from build123d import *

# Parameters (mm, degrees)
F1_DEPTH = 20
F2_SIZE2 = 9.99999
F2_SIZE  = 9.99999


# Not quite as in the source:
# - a fillet or chamfer is up to 0.001 mm smaller than in the source, because OpenCascade refuses the exact size


with BuildPart() as f1:
    # F0 (on Top) → F1 (new body)
    with BuildSketch(Plane.XY):
        Polygon((-50.6066017178, 10.6066017178), (-40, 0), (-40, -79.367487377), (40, -79.367487377), (40, 0), (50.6066017178, 10.6066017178), (0, 61.2132034356), align=None)
        Polygon((40, -79.367487377), (-40, -79.367487377), (-40, -158.7349747541), (-50.6066017178, -169.3415764719), (0, -219.9481781897), (50.6066017178, -169.3415764719), (40, -158.7349747541), align=None)
    extrude(amount=F1_DEPTH)

    # F2 (size 10 and 10 in the source; OpenCascade refuses exactly that, so slightly less here)
    f2_edges = [f1.edges().sort_by_distance(p)[0] for p in [
        (40, -79.367487, 20),
        (25.303301, 35.909903, 20),
        (-25.303301, 35.909903, 20),
        (-45.303301, 5.303301, 20),
        (45.303301, 5.303301, 20),
        (-40, -79.367487, 20),
        (-45.303301, -164.038276, 20),
        (-25.303301, -194.644877, 20),
        (25.303301, -194.644877, 20),
        (45.303301, -164.038276, 20),
        (40, -79.367487, 0),
        (25.303301, -194.644877, 0),
        (45.303301, -164.038276, 0),
        (-25.303301, -194.644877, 0),
        (-45.303301, -164.038276, 0),
        (-40, -79.367487, 0),
        (-45.303301, 5.303301, 0),
        (-25.303301, 35.909903, 0),
    ]]
    chamfer(f2_edges, length=F2_SIZE, length2=F2_SIZE2)


solid = f1.part
Check sheet for the modelled part. Datum: model origin and axes. Units: mm. A direction names the side the tool comes from. Round coordinates to 2 decimals unless told otherwise and drop trailing zeros. Loops run counter-clockwise (first coordinate to the right, second up) from the corner with the lowest first, then second, coordinate; pieces in that order, holes last. Notation, with made-up numbers: (68, -13) - (108, -13) arc R36 cw to (108, 26) - close; hole circle Ø8 at (15, 87). An arc over 180 degrees is marked (long way). Answer as CSV lines item,"result". Start each with the question number.
Item 1: Section check B-B (z = 14). Record the boundary of the cut face in (x, y), and give its area (3 significant figures).
Item 2: Depth check by flat-ended pin: P1, Ø4, axis at y = -3.5, z = 7, coming from the -X side; P2, Ø2, axis at x = -14, z = 15, coming from the -Y side; P3, Ø1, axis at x = -4, z = 11, coming from the -Y side. Enter the tip coordinate at first touch or a pass-through.
Item 3: Set-up check for faces 1 (the flat face through (-40.159, -166.064, 15.07)), 2 (the flat face through (-38.84, 6.01, 4.93)), 3 (the flat face through (35, -81, 15)): record each of +Z, -Z, +X, -X, +Y, -Y from which the full face is reachable in a straight line by a thin tool's end or side.
Item 4: Scan lines: line 1 (Y direction, x = 42.5, z = 9.5); line 2 (Y direction, x = -19, z = 2.5); line 3 (Z direction, x = 30.5, y = -120). Record each from-to range of solid material in increasing order. Write a range as [from, to].
Report:
1,outline,"(-44.95, -169.34) - (0, -214.29) - (44.95, -169.34) - (36, -160.39) - (36, 1.66) - (44.95, 10.61) - (0, 55.56) - (-44.95, 10.61) - (-36, 1.66) - (-36, -160.39) - close"
1,area,"17,200 mm2"
2,P1,"stops at x = -39"
2,P2,"stops at y = -200.61"
2,P3,"stops at y = -215.4"
3,face 1,"+Z, -X"
3,face 2,"-Z, -X"
3,face 3,"+Z, +X"
4,line 1,"y = [-176.74, -161.94], [2.5, 18.71]"
4,line 2,"y = [-190.34, 31.61]"
4,line 3,"z = [0.5, 19.5]"
